from build123d import *

# Parameters (mm, degrees)
F1_DEPTH  = 2.5
F2_W      = 8
F2_H      = 1.5
F3_DEPTH  = 6.5
F4_R      = 0.5
F5_DEPTH  = 25
F6_W      = 0.8
F6_H      = 3
F7_DEPTH  = 3.1
F8_W      = 1
F8_H      = 3
F9_DEPTH  = 1
F11_DEPTH = 0.8
F13_DEPTH = 3
F15_DEPTH = 7
F16_R     = 4
F17_DEPTH = 2.9
F18_R     = 4
F19_DEPTH = 2.9
F20_R     = 3.5
F21_DEPTH = 25
F23_DEPTH = 25


with BuildPart() as f1:
    # F0 (on Right) → F1 (new body)
    with BuildSketch(Plane.YZ):
        with BuildLine():
            Line((11, 5), (-11, 5))
            ThreePointArc((-11, 5), (-14.535534, 3.535534), (-16, 0))
            ThreePointArc((-16, 0), (-14.535534, -3.535534), (-11, -5))
            Line((-11, -5), (11, -5))
            ThreePointArc((11, -5), (14.535534, -3.535534), (16, 0))
            ThreePointArc((16, 0), (14.535534, 3.535534), (11, 5))
        make_face()
    extrude(amount=F1_DEPTH)

    # F2 (on face) → F3 (join)
    with BuildSketch(Plane.YZ.offset(2.5)):
        with Locations((3, 2.25)):
            Rectangle(F2_W, F2_H)
        with Locations((3, -2.25)):
            Rectangle(F2_W, F2_H)
    extrude(amount=F3_DEPTH)

    # F4 (on face) → F5 (cut)
    with BuildSketch(Plane(origin=(0, 0, -3), x_dir=(1, 0, 0), z_dir=(0, 0, -1))):
        with BuildLine():
            Line((9, -6), (9, -3))
            ThreePointArc((9, -3), (8.12132, -5.12132), (6, -6))
            Line((6, -6), (3.575691, -6))
            ThreePointArc((3.575691, -6), (2.879031, -6.329165), (2.5, -7))
            Line((2.5, -7), (9, -7))
            Line((9, -7), (9, -6))
        make_face()
        with BuildLine():
            Line((9, 1), (2.5, 1))
            ThreePointArc((2.5, 1), (2.854094, 0.30234), (3.575691, 0))
            Line((3.575691, 0), (6, 0))
            ThreePointArc((6, 0), (8.12132, -0.87868), (9, -3))
            Line((9, -3), (9, 0))
            Line((9, 0), (9, 1))
        make_face()
        with Locations((6, -3)):
            Circle(F4_R)
    extrude(amount=-F5_DEPTH, mode=Mode.SUBTRACT)

    # F6 (on face) → F7 (join)
    with BuildSketch(Plane.YZ.offset(2.5)):
        with Locations((0.4, 0)):
            Rectangle(F6_W, F6_H)
        Polygon((5.2, 1.5), (5.2, 1.4), (5.2, -0.5), (6, -0.5), (6, 1.5), align=None)
    extrude(amount=F7_DEPTH)

    # F8 (on face) → F9 (join)
    with BuildSketch(Plane.YZ.offset(2.5)):
        with BuildLine():
            Line((13, -1.999869), (13, -2))
            Line((13, -2), (11, -2))
            Line((11, -2), (10, -2))
            Line((10, -2), (10, -3))
            Line((10, -3), (13, -3))
            ThreePointArc((13, -3), (13.701444, -2.712777), (14, -2.016082))
            Line((14, -2.016082), (14, 1))
            Line((14, 1), (13, 1))
            Line((13, 1), (13, 0))
            Line((13, 0), (13, -1.999869))
        make_face()
        with Locations((2.868138, 0)):
            Rectangle(F8_W, F8_H)
    extrude(amount=F9_DEPTH)

    # F10 (on face) → F11 (join)
    with BuildSketch(Plane.YZ.offset(2.5)):
        Polygon((-9.4, -4), (-8.9, -4), (-8.4, -4), (-8.4, 4), (-8.9, 4), (-9.4, 4), align=None)
        with BuildLine():
            Line((-12, -4), (-12, 0))
            Line((-12, 0), (-12, 4))
            ThreePointArc((-12, 4), (-12.692073, 3.722199), (-13, 3.042993))
            Line((-13, 3.042993), (-13, -3.125271))
            ThreePointArc((-13, -3.125271), (-12.664295, -3.750459), (-12, -4))
        make_face()
    extrude(amount=F11_DEPTH)

    # F12 (on face) → F13 (join)
    with BuildSketch(Plane(origin=(0, 0, 0), x_dir=(0, -1, 0), z_dir=(-1, 0, 0))):
        Polygon((-6, 3), (-6, 0), (-6, -3), (0, -3), (0, 3), align=None)
    extrude(amount=F13_DEPTH)

    # F14 (on face) → F15 (join)
    with BuildSketch(Plane(origin=(-3, 0, 0), x_dir=(0, -1, 0), z_dir=(-1, 0, 0))):
        Polygon((-9, -3), (-6, -3), (3, -3), (3, 3), (0, 3), (-9, 3), align=None)
    extrude(amount=F15_DEPTH)

    # F16 (on face) → F17 (cut)
    with BuildSketch(Plane(origin=(0, 0, -3), x_dir=(1, 0, 0), z_dir=(0, 0, -1))):
        with Locations((-7.8, -3)):
            Circle(F16_R)
    extrude(amount=-F17_DEPTH, mode=Mode.SUBTRACT)

    # F18 (on face) → F19 (cut)
    with BuildSketch(Plane.XY.offset(3)):
        with Locations((-7.8, 3)):
            Circle(F18_R)
    extrude(amount=-F19_DEPTH, mode=Mode.SUBTRACT)

    # F20 (on face) → F21 (cut)
    with BuildSketch(Plane.XY.offset(0.1)):
        with Locations((-7.8, 3)):
            Circle(F20_R)
    extrude(amount=-F21_DEPTH, mode=Mode.SUBTRACT)

    # F22 (on face) → F23 (cut)
    with BuildSketch(Plane.XY.offset(3)):
        with BuildLine():
            ThreePointArc((-12.6, 6.6), (-7.8, 9), (-3, 6.6))
            Line((-3, 6.6), (-3, 10.6))
            Line((-3, 10.6), (-18.027099, 10.6))
            Line((-18.027099, 10.6), (-18.027099, -4.6))
            Line((-18.027099, -4.6), (-3, -4.6))
            Line((-3, -4.6), (-3, -0.6))
            ThreePointArc((-3, -0.6), (-7.8, -3), (-12.6, -0.6))
            Line((-12.6, -0.6), (-7.874562, -0.6))
            Line((-7.874562, -0.6), (-7.874562, 6.6))
            Line((-7.874562, 6.6), (-12.6, 6.6))
        make_face()
    extrude(amount=-F23_DEPTH, mode=Mode.SUBTRACT)


solid = f1.part
Work out the finished part from the listing and answer in its coordinate system (mm). A direction names the side the tool comes from. Round coordinates to 2 decimals unless told otherwise and drop trailing zeros. Order: outer loops, then holes, each group sorted by start corner. A loop starts at its lowest first (then second) coordinate and runs counter-clockwise, first axis right, second up. Notation, with made-up numbers: M 81.25,-5.5 L 139.25,-5.5 A10 ccw 139.25,10.5 Z; hole C 79.25,67 d4. An arc over 180 degrees is marked long. Put each result on its own line as item: value. Start each with the question number.
Q1. Section A-A, the plane x = 7.75 is taken. Write down the section's boundary in (y, z), and give its area (3 significant figures).
Q2. Section C-C, the plane y = 12.5 is taken. Write down the section's boundary in (x, z).
Q3. Flat-ended cylindrical pins translate along their axes: pin 1 (5 mm diameter, centred on x = 3, z = 3, fed in from +Y); pin 2 (1 mm diameter, centred on x = 6.5, y = 6, fed in from +Z); pin 3 (11 mm diameter, centred on x = -6, y = 2.5, fed in from -Z); pin 4 (1 mm diameter, centred on x = 4.5, y = -11, fed in from +Z). Find the tip coordinate at first contact, or state that the pin passes through.
Q4. Straight lines are drawn through the part: L1, parallel to Y at x = -7.8, z = -1; L2, parallel to X at y = 3, z = 2.2; L3, parallel to Y at x = 6, z = -2.3. For each, find the intervals that lie inside material, in ascending order. Write a range as [from, to].
Q5. For a pull along Y with two mould halves and no side action, classify faces 1 (the cylindrical face through (2.846, -0.31, -2.26)), 2 (the cylindrical face through (-6.113, -2.758, 0.042)), 3 (the cylindrical face through (2.993, 13.694, -2.72)) as pulls with the +Y half, pulls with the -Y half, needs draft (parallel to the pull), parting line crosses it, or undercut.
Q6. A tool of negligible diameter and unlimited length cuts with its end or side. For faces 4 (the flat face through (-9.7, 6.6, 0.2)), 5 (the cylindrical face through (2.846, -0.31, 2.239)), 6 (the flat face through (-1, 6, 0)), 7 (the flat face through (-4, 3, 0.1)), 8 (the flat face through (-1, 0, 0)), from which of +Z, -Z, +X, -X, +Y, -Y can it reach the whole face along a straight path? Write none if from no direction.
Q7. Section D-D, the plane y = -6 is taken. Write down the section's boundary in (x, z).
Findings below:
1. outline: M 0.56,-3 L 5.44,-3 L 5.44,-1.5 L 0.56,-1.5 Z; M 0.56,1.5 L 5.44,1.5 L 5.44,3 L 0.56,3 Z
1. area: 14.6 mm^2
2. outline: M 0,-4.77 L 2.5,-4.77 L 2.5,-3 L 3.5,-3 L 3.5,-2 L 2.5,-2 L 2.5,4.77 L 0,4.77 Z
3. pin 1: stops at y = 15.97
3. pin 2: stops at z = 3
3. pin 3: stops at z = -3
3. pin 4: passes through
4. L1: y = [-3, -1], [7, 9]
4. L2: x = [-3.8, 5.5], [6.5, 9]
4. L3: y = [0, 2.5], [3.5, 6]
5. face 1: undercut
5. face 2: pulls with the -Y half
5. face 3: pulls with the +Y half
6. face 4: +Z, -Z, -X
6. face 5: +Z, -Z, +X
6. face 6: +Z, -Z, +Y
6. face 7: +Z
6. face 8: +Z, -Z, -Y
7. outline: M 0,-5 L 2.5,-5 L 2.5,5 L 0,5 Z
